Verification items for the finished model (mm, model axes). Face numbers are marked on the shaded views. A direction names the side the tool comes from. Give positions to 0.01 mm unless a question says otherwise; leave off trailing zeros. Order: outer loops, then holes, each group sorted by start corner. A loop starts at its lowest first (then second) coordinate and runs counter-clockwise, first axis right, second up. Notation, with made-up numbers: M 6,16.5 L 46,16.5 A26 ccw 46,55.5 Z; hole C 11,43.5 d3. An arc over 180 degrees is marked long. Answer as a JSON object with one key per item and string values.
```python
from build123d import *

# Parameters (mm, degrees)
EXTRUDE_START   = 13
SKETCH_1_W      = 30.8
SKETCH_1_H      = 30.8
EXTRUDE_1_DEPTH = 75
SKETCH_3_W      = 43.086164537
SKETCH_3_H      = 5
EXTRUDE_2_DEPTH = 40.6


with BuildPart() as part:
    # ｽｹｯﾁ1 → ﾎﾞｽ - 押し出し1 (new body)
    with BuildSketch(Plane.XY.offset(EXTRUDE_START)):
        with Locations((56, 18.4)):
            Rectangle(SKETCH_1_W, SKETCH_1_H)
        Polygon((53.6, 26.002672003), (53.6, 28.8), (45.6, 28.8), (45.6, 20.8), (48.397327997, 20.8), (48.397327997, 23.6), (48.797327997, 23.6), (51.597327997, 20.8), (51.597327997, 16), (48.797327997, 13.2), (48.397327997, 13.2), (48.397327997, 16), (45.6, 16), (45.6, 8), (53.6, 8), (53.6, 10.797327997), (50.8, 10.797327997), (50.8, 11.197327997), (53.6, 13.997327997), (58.4, 13.997327997), (61.2, 11.197327997), (61.2, 10.797327997), (58.4, 10.797327997), (58.4, 8), (66.4, 8), (66.4, 16), (63.602672003, 16), (63.602672003, 13.2), (63.202672003, 13.2), (60.402672003, 16), (60.402672003, 20.8), (63.202672003, 23.6), (63.602672003, 23.6), (63.602672003, 20.8), (66.4, 20.8), (66.4, 28.8), (58.4, 28.8), (58.4, 26.002672003), (61.2, 26.002672003), (61.2, 25.602672003), (58.4, 22.802672003), (53.6, 22.802672003), (50.8, 25.602672003), (50.8, 26.002672003), align=None, mode=Mode.SUBTRACT)
    extrude(amount=EXTRUDE_1_DEPTH)

    # ｽｹｯﾁ3 → ﾎﾞｽ - 押し出し2 (add)
    with BuildSketch(Plane.ZY.offset(-40.6)):
        with Locations((43.543082269, 5.5)):
            Rectangle(SKETCH_3_W, SKETCH_3_H)
    extrude(amount=EXTRUDE_2_DEPTH)


solid = part.part
```
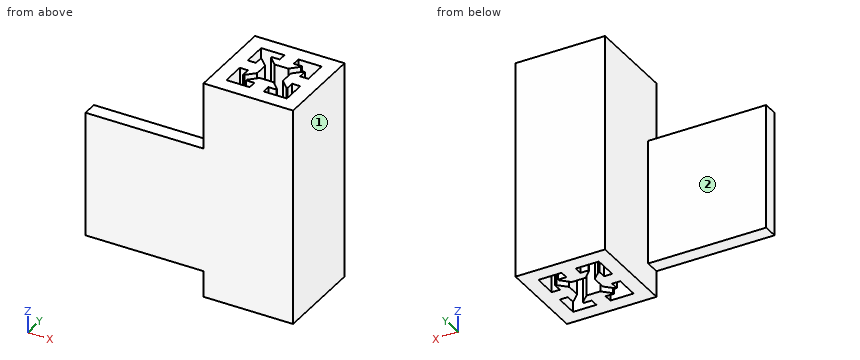
Q1. Section check C-C on y = 6. Record the cut outline in (x, z).
Resolved:
{"outline": "M 0,22 L 40.6,22 L 40.6,13 L 71.4,13 L 71.4,88 L 40.6,88 L 40.6,65.09 L 0,65.09 Z"}
Q2. Section check D-D on x = 30. Record the cut outline in (y, z), then the cut area to 3 significant figures.
Resolved:
{"outline": "M 3,22 L 8,22 L 8,65.09 L 3,65.09 Z", "area": "215 mm²"}
Q3. Tool access check on the marked faces 1 and 2. Record the directions out of +Z, -Z, +X, -X, +Y, -Y that give a thin tool (end or side, any length) a straight path to the whole face; none if there is none.
Resolved:
{"face 1": "+Z, -Z, +X, +Y, -Y", "face 2": "+Z, -Z, -X, +Y"}
Q4. Gauge pin test, flat end, axial feed: pin 1 Ø1.4 at (y, z) = (10, 34.5) entering from -X. Record the tip position at first contact, or that the pin passes through.
Resolved:
{"pin 1": "stops at x = 40.6"}
Q5. Section check B-B on y = 19.5. Record the cut outline in (x, z).
Resolved:
{"outline": "M 40.6,13 L 51.6,13 L 51.6,88 L 40.6,88 Z; M 60.4,13 L 71.4,13 L 71.4,88 L 60.4,88 Z"}
Q6. Section check A-A on x = 55.5. Record the cut outline in (y, z), then the cut area to 3 significant figures.
Resolved:
{"outline": "M 3,13 L 14,13 L 14,88 L 3,88 Z; M 22.8,13 L 33.8,13 L 33.8,88 L 22.8,88 Z", "area": "1,650 mm²"}
Q7. Material ranges on L1, parallel to X at y = 27, z = 33; L2, parallel to X at y = 19, z = 74; L3, parallel to Y at x = 56, z = 70, recorded low to high.
Resolved:
{"L1": "x = 40.6 to 45.6, 53.6 to 58.4, 66.4 to 71.4", "L2": "x = 40.6 to 51.6, 60.4 to 71.4", "L3": "y = 3 to 14, 22.8 to 33.8"}
